Check sheet for the modelled part. Datum: model origin and axes. Units: mm. A direction names the side the tool comes from. Give positions to 0.01 mm unless a question says otherwise; leave off trailing zeros. Order: outer loops, then holes, each group sorted by start corner. A loop starts at its lowest first (then second) coordinate and runs counter-clockwise, first axis right, second up. Notation, with made-up numbers: (32, 6) -> (37, 6) arc R24 cw to (37, 21) -> close; hole circle Ø4 at (23, -10.75). An arc over 180 degrees is marked (long way). Answer in a Markdown table with one row per item. Add a question column.
(1) Cross-section at B-B (z = 0). Record the cut outline in (x, y), then the cut area to 3 significant figures.
(2) Cross-section at D-D (y = 4.45). Record the cut outline in (x, z), then the cut area to 3 significant figures.
(3) Cross-section at C-C (z = -13.25). Record the cut outline in (x, y).
(4) Thickness scan on L1, parallel to X at y = 3.45, z = 0; L2, parallel to Z at x = -2.75, y = 4.8; L3, parallel to X at y = 4.6, z = 0. Record the ranges inside material, lowest first. Write a range as [from, to].
(5) Go/stop test with flat-tipped pins: pin 1 (2 mm diameter, centred on x = 0, z = 0, fed in from +Y); pin 2 (3 mm diameter, centred on x = 9, y = 5, fed in from +Z). Record where each tip stops, or that it passes through.
(6) Set-up check for faces 1 (the face through (0.66, 4.986, -14.985)), 2 (the face through (12.3, 2, -0.1)), 3 (the face through (0, 0, 3)), 4 (the face through (1, 3, 1)), 5 (the face through (-3.955, 5.014, -5.158)): record each of +Z, -Z, +X, -X, +Y, -Y from which the full face is reachable in a straight line by a thin tool's end or side.
(7) Release check for a two-part mould opening along X. For faces 6 (the face through (-3, 6, 6)), 7 (the face through (3.604, 2.986, 11.446)), 8 (the face through (-2.44, 1.48, 0.54)) record: released by +X, released by -X, zero draft, split by the parting line, or undercut.
(8) Cross-section at A-A (x = 0). State how many separate pieces and enclosed holes the cut face has, then the cut area to 3 significant figures.
```python
from build123d import *

# Parameters (mm, degrees)
SKETCH1_R           = 15
BOSS_EXTRUDE1_DEPTH = 2
SKETCH2_R           = 12
BOSS_EXTRUDE2_DEPTH = 2
SKETCH3_R           = 15
BOSS_EXTRUDE3_DEPTH = 2
SKETCH6_R           = 2.5
CUT_EXTRUDE5_DEPTH  = 3
SKETCH4_R           = 6.5
CUT_EXTRUDE6_DEPTH  = 2
SKETCH10_R          = 0.8
CUT_EXTRUDE7_DEPTH  = 22.587033145
SKETCH11_R          = 1
CUT_EXTRUDE8_DEPTH  = 23.045407685


with BuildPart() as part:
    # Sketch1 → Boss-Extrude1 (new body)
    with BuildSketch(Plane(origin=(0, 0, 0), x_dir=(1, 0, 0), z_dir=(0, 1, 0))):
        with Locations(Location((0, 0, 0), (0, 0, 270))):
            Circle(SKETCH1_R)
    extrude(amount=BOSS_EXTRUDE1_DEPTH)

    # Sketch2 → Boss-Extrude2 (add)
    with BuildSketch(Plane(origin=(0, 2, 0), x_dir=(1, 0, 0), z_dir=(0, 1, 0))):
        with Locations(Location((0, 0, 0), (0, 0, 270))):
            Circle(SKETCH2_R)
    extrude(amount=BOSS_EXTRUDE2_DEPTH)

    # Sketch3 → Boss-Extrude3 (add)
    with BuildSketch(Plane(origin=(0, 4, 0), x_dir=(1, 0, 0), z_dir=(0, 1, 0))):
        with Locations(Location((0, 0, 0), (0, 0, 270))):
            Circle(SKETCH3_R)
    extrude(amount=BOSS_EXTRUDE3_DEPTH)

    # Sketch6 → Cut-Extrude5 (cut)
    with BuildSketch(Plane.XZ):
        with Locations(Location((0, 0, 0), (0, 0, 270))):
            Circle(SKETCH6_R)
    extrude(amount=-CUT_EXTRUDE5_DEPTH, mode=Mode.SUBTRACT)

    # Sketch4 → Cut-Extrude6 (cut)
    with BuildSketch(Plane(origin=(0, 6, 0), x_dir=(1, 0, 0), z_dir=(0, 1, 0))):
        with Locations(Location((0, 0, 0), (0, 0, 270))):
            Circle(SKETCH4_R)
    extrude(amount=-CUT_EXTRUDE6_DEPTH, mode=Mode.SUBTRACT)

    # Sketch10 → Cut-Extrude7 (cut, through all)
    with BuildSketch(Plane(origin=(0, 4, 0), x_dir=(1, 0, 0), z_dir=(0, 1, 0))):
        with Locations(Location((0, 0, 0), (0, 0, 270))):
            Circle(SKETCH10_R)
    extrude(amount=-CUT_EXTRUDE7_DEPTH, mode=Mode.SUBTRACT)

    # Sketch11 → Cut-Extrude8 (cut, through all)
    with BuildSketch(Plane(origin=(0, 6, 0), x_dir=(1, 0, 0), z_dir=(0, 1, 0))):
        with Locations(Location((0, 13.25, 0), (0, 0, 270))):
            Circle(SKETCH11_R)
        with Locations(Location((-2.5, 13.01201368, 0), (0, 0, 270))):
            Circle(SKETCH11_R)
    extrude(amount=-CUT_EXTRUDE8_DEPTH, mode=Mode.SUBTRACT)


solid = part.part
```
Answer below:
| question | item | result |
|---|---|---|
| 1 | outline | (-15, 0) -> (-2.5, 0) -> (-2.5, 3) -> (-0.8, 3) -> (-0.8, 4) -> (-6.5, 4) -> (-6.5, 6) -> (-15, 6) -> (-15, 4) -> (-12, 4) -> (-12, 2) -> (-15, 2) -> close; (0.8, 3) -> (2.5, 3) -> (2.5, 0) -> (15, 0) -> (15, 2) -> (12, 2) -> (12, 4) -> (15, 4) -> (15, 6) -> (6.5, 6) -> (6.5, 4) -> (0.8, 4) -> close |
| 1 | area | 125 mm² |
| 2 | outline | circle Ø30 at (0, 0); hole circle Ø13 at (0, 0); hole circle Ø2 at (-2.5, -13.01); hole circle Ø2 at (0, -13.25) |
| 2 | area | 568 mm² |
| 3 | outline | (-7.03, 0) -> (-3.47, 0) -> (-3.47, 2) -> (-7.03, 2) -> close; (-7.03, 4) -> (-3.47, 4) -> (-3.47, 6) -> (-7.03, 6) -> close; (-1.53, 0) -> (-1, 0) -> (-1, 2) -> (-1.53, 2) -> close; (-1.53, 4) -> (-1, 4) -> (-1, 6) -> (-1.53, 6) -> close; (1, 0) -> (7.03, 0) -> (7.03, 2) -> (1, 2) -> close; (1, 4) -> (7.03, 4) -> (7.03, 6) -> (1, 6) -> close |
| 4 | L1 | x = [-12, -0.8], [0.8, 12] |
| 4 | L2 | z = [-14.75, -13.98], [-12.04, -5.89], [5.89, 14.75] |
| 4 | L3 | x = [-15, -6.5], [6.5, 15] |
| 5 | pin 1 | stops at y = 4 |
| 5 | pin 2 | stops at z = 12.99 |
| 6 | face 1 | +Y, -Y |
| 6 | face 2 | none |
| 6 | face 3 | +Z, -Z, +X, -X, -Y |
| 6 | face 4 | -Y |
| 6 | face 5 | +Y |
| 7 | face 6 | zero draft |
| 7 | face 7 | split by the parting line |
| 7 | face 8 | undercut |
| 8 | separate pieces | 4 |
| 8 | enclosed holes | 0 |
| 8 | area | 117 mm² |
